```python
from build123d import *

# Parameters (mm, degrees)
BOSS_EXTRUDE3_DEPTH = 7.8
SKETCH2_R           = 2.4
CUT_EXTRUDE6_DEPTH  = 7.8
SKETCH3_R           = 3.05
CUT_EXTRUDE7_DEPTH  = 0.8
SKETCH4_R           = 3.05
CUT_EXTRUDE8_DEPTH  = 0.8


with BuildPart() as part:
    # Sketch1 → Boss-Extrude3 (new body)
    with BuildSketch(Plane(origin=(0, 0, 0), x_dir=(1, 0, 0), z_dir=(0, 1, 0))):
        with BuildLine():
            Line((-16, 3.7), (-8, 3.7))
            ThreePointArc((-8, 3.7), (-4.3, 0), (-8, -3.7))
            Line((-8, -3.7), (-16, -3.7))
            ThreePointArc((-16, -3.7), (-19.7, 0), (-16, 3.7))
        make_face()
    extrude(amount=BOSS_EXTRUDE3_DEPTH)

    # Sketch2 → Cut-Extrude6 (cut)
    with BuildSketch(Plane(origin=(0, 7.8, 0), x_dir=(1, 0, 0), z_dir=(0, 1, 0))):
        with Locations((-16, 0)):
            Circle(SKETCH2_R)
        with Locations((-8, 0)):
            Circle(SKETCH2_R)
    extrude(amount=-CUT_EXTRUDE6_DEPTH, mode=Mode.SUBTRACT)

    # Sketch3 → Cut-Extrude7 (cut)
    with BuildSketch(Plane(origin=(0, 7.8, 0), x_dir=(1, 0, 0), z_dir=(0, 1, 0))):
        with Locations((-16, 0)):
            Circle(SKETCH3_R)
        with Locations((-8, 0)):
            Circle(SKETCH3_R)
    extrude(amount=-CUT_EXTRUDE7_DEPTH, mode=Mode.SUBTRACT)

    # Sketch4 → Cut-Extrude8 (cut)
    with BuildSketch(Plane.XZ):
        with Locations((-16, 0)):
            Circle(SKETCH4_R)
        with Locations((-8, 0)):
            Circle(SKETCH4_R)
    extrude(amount=-CUT_EXTRUDE8_DEPTH, mode=Mode.SUBTRACT)


solid = part.part
```
The listing builds one solid part. Answer for the finished solid, in the listing's coordinates (mm). A direction names the side the tool comes from. Round coordinates to 2 decimals unless told otherwise and drop trailing zeros. Write each loop counter-clockwise with the first axis right and the second up, starting at its lowest first coordinate (ties: lowest second). Pieces come first, ordered by that corner, then holes. Notation, with made-up numbers: (62, 28) -> (103, 28) arc R17 ccw to (103, 57) -> close; hole circle Ø6 at (83.25, -11.75). An arc over 180 degrees is marked (long way). Use CSV: the item, a comma, the result in double quotes. Start each with the question number.
(1) Consider L1, parallel to X at y = 4, z = 0; L2, parallel to X at y = 7.4, z = 0; L3, parallel to Z at x = -16, y = 2.25. Determine where each line is inside the solid, lowest interval first. Write a range as from..to.
(2) Section C-C on x = -14.5 is taken. Give the vertices of the cut face in (y, z).
(3) Which of the six approach directions +Z, -Z, +X, -X, +Y, -Y give full straight-line access (tool end or side, diameter ignored) to faces 4 (the face through (-13.09, 7.41, -0.92)), 5 (the face through (-18.398, 3.943, -0.106)), 6 (the face through (-10, 0.8, -2))?
(4) Section A-A on z = 0 is taken. Give the vertices of the cut face in (x, y), then the cut area to 3 significant figures.
(5) The mould has two halves that part along X. Classify faces 1 (the face through (-19.7, 3.8, 0.1)), 2 (the face through (-12, 7.8, 0)), 3 (the face through (-11.047, 7.406, -0.134)): released by +X, released by -X, zero draft, split by the parting line, or undercut.
(6) Section B-B on y = 5.5 is taken. Give the vertices of the cut face in (x, z), then the cut area to 3 significant figures.
(7) Section D-D on z = 2 is taken. Give the vertices of the cut face in (x, y), then the cut area to 3 significant figures.
(8) This flat-tipped pin is pushed along its axis until it touches: pin 1 (3 mm diameter, centred on x = -15.5, z = 0.5, fed in from +Y). Where does it stop, or does it pass through?
A:
1,L1,"x = -19.7..-18.4, -13.6..-10.4, -5.6..-4.3"
1,L2,"x = -19.7..-19.05, -12.95..-11.05, -4.95..-4.3"
1,L3,"z = -3.7..-2.4, 2.4..3.7"
2,outline,"(0, -3.7) -> (7.8, -3.7) -> (7.8, -2.66) -> (7, -2.66) -> (7, -1.87) -> (0.8, -1.87) -> (0.8, -2.66) -> (0, -2.66) -> close; (0, 2.66) -> (0.8, 2.66) -> (0.8, 1.87) -> (7, 1.87) -> (7, 2.66) -> (7.8, 2.66) -> (7.8, 3.7) -> (0, 3.7) -> close"
3,face 4,"+Y"
3,face 5,"+Y, -Y"
3,face 6,"-Y"
4,outline,"(-19.7, 0) -> (-19.05, 0) -> (-19.05, 0.8) -> (-18.4, 0.8) -> (-18.4, 7) -> (-19.05, 7) -> (-19.05, 7.8) -> (-19.7, 7.8) -> close; (-13.6, 0.8) -> (-12.95, 0.8) -> (-12.95, 0) -> (-11.05, 0) -> (-11.05, 0.8) -> (-10.4, 0.8) -> (-10.4, 7) -> (-11.05, 7) -> (-11.05, 7.8) -> (-12.95, 7.8) -> (-12.95, 7) -> (-13.6, 7) -> close; (-5.6, 0.8) -> (-4.95, 0.8) -> (-4.95, 0) -> (-4.3, 0) -> (-4.3, 7.8) -> (-4.95, 7.8) -> (-4.95, 7) -> (-5.6, 7) -> close"
4,area,"41.1 mm²"
5,face 1,"released by -X"
5,face 2,"zero draft"
5,face 3,"undercut"
6,outline,"(-16, -3.7) -> (-8, -3.7) arc R3.7 ccw to (-8, 3.7) -> (-16, 3.7) arc R3.7 ccw to start; hole circle Ø4.8 at (-16, 0); hole circle Ø4.8 at (-8, 0)"
6,area,"66.0 mm²"
7,outline,"(-19.11, 0) -> (-18.3, 0) -> (-18.3, 0.8) -> (-17.33, 0.8) -> (-17.33, 7) -> (-18.3, 7) -> (-18.3, 7.8) -> (-19.11, 7.8) -> close; (-14.67, 0.8) -> (-13.7, 0.8) -> (-13.7, 0) -> (-10.3, 0) -> (-10.3, 0.8) -> (-9.33, 0.8) -> (-9.33, 7) -> (-10.3, 7) -> (-10.3, 7.8) -> (-13.7, 7.8) -> (-13.7, 7) -> (-14.67, 7) -> close; (-6.67, 0.8) -> (-5.7, 0.8) -> (-5.7, 0) -> (-4.89, 0) -> (-4.89, 7.8) -> (-5.7, 7.8) -> (-5.7, 7) -> (-6.67, 7) -> close"
7,area,"63.3 mm²"
8,pin 1,"passes through"
